```python
from build123d import *

# Parameters (mm, degrees)
F0_W     = 88.9000000224
F0_H     = 165.1000027703
F1_DEPTH = 12.7
F2_DEPTH = 25.4
F3_DEPTH = 63.5
F4_R     = 6.34999
F5_SIZE2 = 7.332338
F5_SIZE  = 12.69999


# Not quite as in the source:
# - a fillet or chamfer is up to 0.001 mm smaller than in the source, because OpenCascade refuses the exact size


with BuildPart() as f1:
    # F0 (on Top) → F1 (new body)
    with BuildSketch(Plane.XY):
        with Locations((38.1000000112, -1.3851e-06)):
            Rectangle(F0_W, F0_H)
        Polygon((0, 38.1), (0, 76.2), (38.1, 76.2), (76.2, 76.2), (76.2, -38.1), (76.2, -76.2), (38.1, -76.2), (0, -76.2), align=None, mode=Mode.SUBTRACT)
    extrude(amount=F1_DEPTH)

    # F0 (on Top) → F2 (join)
    with BuildSketch(Plane.XY):
        with BuildLine():
            Line((25.4, 38.1), (0, 38.1))
            Line((0, 38.1), (0, -76.2))
            Line((0, -76.2), (38.1, -76.2))
            Line((38.1, -76.2), (38.1, -50.8))
            ThreePointArc((38.1, -50.8), (41.8197438789, -41.8197438789), (50.8, -38.1))
            Line((50.8, -38.1), (76.2, -38.1))
            Line((76.2, -38.1), (76.2, 76.2))
            Line((76.2, 76.2), (38.1, 76.2))
            Line((38.1, 76.2), (38.1, 50.8))
            ThreePointArc((38.1, 50.8), (34.3802561211, 41.8197438789), (25.4, 38.1))
        make_face()
    extrude(amount=F2_DEPTH)

    # F0 (on Top) → F3 (join)
    with BuildSketch(Plane.XY):
        with BuildLine():
            Line((38.1, 76.2), (0, 76.2))
            Line((0, 76.2), (0, 38.1))
            Line((0, 38.1), (25.4, 38.1))
            ThreePointArc((25.4, 38.1), (34.3802561211, 41.8197438789), (38.1, 50.8))
            Line((38.1, 50.8), (38.1, 76.2))
        make_face()
        with BuildLine():
            Line((38.1, -50.8), (38.1, -76.2))
            Line((38.1, -76.2), (76.2, -76.2))
            Line((76.2, -76.2), (76.2, -38.1))
            Line((76.2, -38.1), (50.8, -38.1))
            ThreePointArc((50.8, -38.1), (41.8197438789, -41.8197438789), (38.1, -50.8))
        make_face()
    extrude(amount=F3_DEPTH)

    # F4 (radius 6.35 in the source; OpenCascade refuses exactly that, so slightly less here)
    f4_edges = [f1.edges().sort_by_distance(p)[0] for p in [
        (-6.35, -1e-06, 12.7),
        (38.1, -82.550003, 12.7),
        (82.55, -1e-06, 12.7),
        (38.1, 82.55, 12.7),
    ]]
    fillet(f4_edges, radius=F4_R)

    # F5 (size 12.7 and 7.3323484187 in the source; OpenCascade refuses exactly that, so slightly less here)
    f5_edges = [f1.edges().sort_by_distance(p)[0] for p in [
        (57.15, 76.2, 25.4),
        (76.2, 19.05, 25.4),
        (0, -19.05, 25.4),
        (19.05, -76.2, 25.4),
        (57.15, -76.2, 63.5),
        (76.2, -57.15, 63.5),
        (19.05, 76.2, 63.5),
        (0, 57.15, 63.5),
    ]]
    chamfer(f5_edges, length=F5_SIZE, length2=F5_SIZE2)


solid = f1.part
```
Geometry check sheet. Reference: the model listing, model coordinates, mm. A direction names the side the tool comes from. Give positions to 0.01 mm unless a question says otherwise; leave off trailing zeros. Order: outer loops, then holes, each group sorted by start corner. A loop starts at its lowest first (then second) coordinate and runs counter-clockwise, first axis right, second up. Notation, with made-up numbers: (85.5, -26.5) - (131.5, -26.5) arc R24 cw to (131.5, -10.5) - close; hole circle Ø11 at (3, 41). An arc over 180 degrees is marked (long way). Answer in a Markdown table with one row per item. Add a question column.
Q1. Cross-section at D-D, the plane z = 22. Enter the section's corners in (x, y).
Q2. Tool access check on faces 1 (the flat face through (0, 57, 30)), 2 (the flat face through (18.78, -72.48, 19.14)), 3 (the flat face through (38.1, 63, 43)), 4 (the flat face through (54, -76.2, 31)). Record the directions out of +Z, -Z, +X, -X, +Y, -Y that give a thin tool (end or side, any length) a straight path to the whole face; none if there is none.
Q3. Gauge pin test, flat ends, axial feed: pin 1 (20.5 mm diameter, centred on y = 64, z = 31.5, fed in from +X); pin 2 (7.5 mm diameter, centred on y = -64.5, z = 29, fed in from -X); pin 3 (8 mm diameter, centred on x = 55, z = 50, fed in from +Y). Record the tip position at first contact, or that the pin passes through.
Q4. Material ranges on probe 1 along Z at (x, y) = (61.5, -7.5); probe 2 along Y at (x, z) = (70.5, 48.5); probe 3 along X at (y, z) = (21, 7), recorded low to high. Write a range as from..to.
Q5. Cross-section at A-A, the plane z = 40. Enter the section's corners in (x, y), then the cut area to 3 significant figures.
Check values:
| question | item | result |
|---|---|---|
| 1 | outline | (0, 38.1) - (5.37, 38.1) - (5.37, -70.83) - (38.1, -70.83) - (38.1, -76.2) - (76.2, -76.2) - (76.2, -38.1) - (70.83, -38.1) - (70.83, 70.83) - (38.1, 70.83) - (38.1, 76.2) - (0, 76.2) - close |
| 2 | face 1 | +Z, -X, +Y, -Y |
| 2 | face 2 | +Z, -X, -Y |
| 2 | face 3 | +Z, +X, +Y |
| 2 | face 4 | +Z, +X, -X, -Y |
| 3 | pin 1 | stops at x = 71.26 |
| 3 | pin 2 | stops at x = 7.25 |
| 3 | pin 3 | stops at y = -38.1 |
| 4 | probe 1 | z = 0..25.4 |
| 4 | probe 2 | y = -76.2..-38.1 |
| 4 | probe 3 | x = -6.32..82.52 |
| 5 | outline | (0, 38.1) - (25.4, 38.1) arc R12.7 ccw to (38.1, 50.8) - (38.1, 76.2) - (0, 76.2) - close; (38.1, -76.2) - (76.2, -76.2) - (76.2, -38.1) - (50.8, -38.1) arc R12.7 ccw to (38.1, -50.8) - close |
| 5 | area | 2,830 mm^2 |
